from build123d import *

# Parameters (mm, degrees)
BOSS_EXTRUDE1_DEPTH            = 3.5
BOSS_EXTRUDE1_DEPTH_BACK       = 3.5
SKETCH3_R                      = 1.25
CUT_EXTRUDE5_DEPTH             = 3.5
BOSS_EXTRUDE2_START            = 0.5
SKETCH5_R                      = 2.25
SKETCH5_R_2                    = 1.25
BOSS_EXTRUDE2_DEPTH            = 0.5
CUT_EXTRUDE6_REACH             = 72.102
SKETCH6_R                      = 1.5
CUT_EXTRUDE6_DIRECTION_2_REACH = 72.102
FILLET1_R                      = 0.01


with BuildPart() as part:
    # Sketch1 → Boss-Extrude1 (new, two sides: drawn at the far end of the back side and taken through both)
    with BuildSketch(Plane.XY.offset(-BOSS_EXTRUDE1_DEPTH_BACK)):
        Polygon((-62.621366216, 18.813688138), (-62.621366216, 30.813688138), (31.378633784, 30.813688138), (31.378633784, 18.813688138), (29.878633784, 18.813688138), (29.878633784, 29.313688138), (-61.121366216, 29.313688138), (-61.121366216, 18.813688138), align=None)
    extrude(amount=BOSS_EXTRUDE1_DEPTH + BOSS_EXTRUDE1_DEPTH_BACK)

    # Sketch3 → Cut-Extrude5 (cut)
    with BuildSketch(Plane(origin=(0, 30.813688138, 0), x_dir=(1, 0, 0), z_dir=(0, 1, 0))):
        with Locations(Location((-15.621366216, 0, 0), (0, 0, 180))):
            Circle(SKETCH3_R)
    extrude(amount=-CUT_EXTRUDE5_DEPTH, mode=Mode.SUBTRACT)

    # Sketch5 → Boss-Extrude2 (add)
    with BuildSketch(Plane(origin=(0, 30.813688138, 0), x_dir=(1, 0, 0), z_dir=(0, 1, 0)).offset(BOSS_EXTRUDE2_START)):
        with Locations(Location((-15.621366216, 0, 0), (0, 0, 180))):
            Circle(SKETCH5_R)
        with Locations(Location((-15.621366216, 0, 0), (0, 0, 180))):
            Circle(SKETCH5_R_2, mode=Mode.SUBTRACT)
    extrude(amount=-BOSS_EXTRUDE2_DEPTH)

    # Cut-Extrude6: up to this face of the body (flat: up to its plane)
    cut_extrude6_end = Plane(part.part.faces().sort_by_distance((31.378633784, 24.813688138, 0))[0])
    # Sketch6 → Cut-Extrude6 (cut, up to the picked face)
    with BuildSketch(Plane(origin=(0, 0, 0), x_dir=(0, 0, -1), z_dir=(1, 0, 0)), mode=Mode.PRIVATE) as cut_extrude6_sk1:
        with Locations(Location((0, 22.813688138, 0), (0, 0, 180))):
            Circle(SKETCH6_R)
    cut_extrude6_tool1 = split(extrude(cut_extrude6_sk1.sketch, amount=CUT_EXTRUDE6_REACH, mode=Mode.PRIVATE), bisect_by=cut_extrude6_end, keep=Keep.BOTH, mode=Mode.PRIVATE)
    add(cut_extrude6_tool1.solids().sort_by(Axis((0, 22.813688, 0), (1, 0, 0)))[0], mode=Mode.SUBTRACT)

    # Cut-Extrude6 direction 2: up to this face of the body (flat: up to its plane)
    cut_extrude6_direction_2_end = Plane(part.part.faces().sort_by_distance((-62.621366216, 24.813688138, 0))[0])
    # Sketch6 → Cut-Extrude6 direction 2 (cut, up to the picked face)
    with BuildSketch(Plane(origin=(0, 0, 0), x_dir=(0, 0, -1), z_dir=(1, 0, 0)), mode=Mode.PRIVATE) as cut_extrude6_direction_2_sk1:
        with Locations(Location((0, 22.813688138, 0), (0, 0, 180))):
            Circle(SKETCH6_R)
    cut_extrude6_direction_2_tool1 = split(extrude(cut_extrude6_direction_2_sk1.sketch, amount=-CUT_EXTRUDE6_DIRECTION_2_REACH, mode=Mode.PRIVATE), bisect_by=cut_extrude6_direction_2_end, keep=Keep.BOTH, mode=Mode.PRIVATE)
    add(cut_extrude6_direction_2_tool1.solids().sort_by(Axis((0, 22.813688, 0), (-1, 0, 0)))[0], mode=Mode.SUBTRACT)

    # Fillet1
    fillet1_edges = [part.edges().sort_by_distance(p)[0] for p in [
        (-15.621366216, 29.313688138, -3.5),
        (-62.621366216, 18.813688138, 0),
        (-62.621366216, 30.813688138, 0),
        (31.378633784, 30.813688138, 0),
        (31.378633784, 18.813688138, 0),
        (29.878633784, 18.813688138, 0),
        (-61.121366216, 29.313688138, 0),
        (-61.121366216, 18.813688138, 0),
        (29.878633784, 24.063688138, -3.5),
        (30.628633784, 18.813688138, -3.5),
        (-61.871366216, 18.813688138, 3.5),
        (-61.121366216, 24.063688138, 3.5),
        (-15.621366216, 29.313688138, 3.5),
        (29.878633784, 24.063688138, 3.5),
        (30.628633784, 18.813688138, 3.5),
        (31.378633784, 24.813688138, -3.5),
        (31.378633784, 24.813688138, 3.5),
        (-15.621366216, 30.813688138, 3.5),
        (-62.621366216, 24.813688138, 3.5),
        (-15.621366216, 30.813688138, -3.5),
        (-62.621366216, 24.813688138, -3.5),
        (-13.371366216, 31.313688138, 0),
        (-14.371366216, 31.313688138, 0),
        (-61.871366216, 18.813688138, -3.5),
        (29.878633784, 22.813688138, -1.5),
        (-61.121366216, 22.813688138, -1.5),
        (-62.621366216, 22.813688138, -1.5),
        (31.378633784, 22.813688138, -1.5),
        (-61.121366216, 24.063688138, -3.5),
    ]]
    fillet(fillet1_edges, radius=FILLET1_R)


solid = part.part
Work out the finished part from the listing and answer in its coordinate system (mm). A direction names the side the tool comes from. Coordinates: 2 decimals unless noted, no trailing zeros. Answer in a Markdown table with one row per item. Add a question column.
1. Consider L1, parallel to Y at x = -62.05, z = 0; L2, parallel to X at y = 27.25, z = -2.5; L3, parallel to Y at x = 23.5, z = -0.25. Determine where each line is inside the solid, lowest interval first.
2. Find section C-C, the plane z = 0. State how many separate pieces and enclosed holes the cut face has, then the cut area to 3 significant figures.
3. Flat-ended cylindrical pins translate along their axes: P1, Ø1, axis at x = 7, z = -2.5, coming from the -Y side; P2, Ø3.5, axis at x = -2.5, z = -1, coming from the +Y side; P3, Ø2.5, axis at y = 22.81, z = 0, coming from the +X side. Find the tip coordinate at first contact, or state that the pin passes through.
4. A tool of negligible diameter and unlimited length cuts with its end or side. For faces 1 (the flat face through (29.879, 25, 0)), 2 (the cylindrical face through (-61.86, 21.55, 0.81)), from which of +Z, -Z, +X, -X, +Y, -Y can it reach the whole face along a straight path? Write none if from no direction.
5. The mould has two halves that part along Z. Classify faces 3 (the cylindrical face through (-13.374, 31.062, 0.099)), 4 (the cylindrical face through (-16.814, 30.323, 0.375)), 5 (the flat face through (-62.621, 25, 0)): pulls with the +Z half, pulls with the -Z half, needs draft (parallel to the pull), parting line crosses it, or undercut.
Reported:
| question | item | result |
|---|---|---|
| 1 | L1 | y = 18.81 to 21.31, 24.31 to 30.81 |
| 1 | L2 | x = -62.62 to -61.12, 29.88 to 31.38 |
| 1 | L3 | y = 29.31 to 30.81 |
| 2 | separate pieces | 4 |
| 2 | enclosed holes | 0 |
| 2 | area | 161 mm^2 |
| 3 | P1 | stops at y = 29.31 |
| 3 | P2 | stops at y = 30.81 |
| 3 | P3 | passes through |
| 4 | face 1 | +Z, -Z, -Y |
| 4 | face 2 | +X, -X |
| 5 | face 3 | parting line crosses it |
| 5 | face 4 | undercut |
| 5 | face 5 | needs draft |
